from build123d import *

# Parameters (mm, degrees)
SKETCH1_W           = 100
SKETCH1_H           = 200
SKETCH1_W_2         = 67
SKETCH1_H_2         = 110
BOSS_EXTRUDE1_DEPTH = 2
SKETCH2_W           = 100
SKETCH2_H           = 200
SKETCH2_W_2         = 94
SKETCH2_H_2         = 194
BOSS_EXTRUDE2_DEPTH = 16.4
SKETCH3_R           = 1.15
BOSS_EXTRUDE3_DEPTH = 2
BOSS_EXTRUDE4_DEPTH = 25
SKETCH8_W           = 100
SKETCH8_H           = 110
BOSS_EXTRUDE5_DEPTH = 3
SKETCH9_W           = 11
SKETCH9_H           = 13
CUT_EXTRUDE2_DEPTH  = 36
SKETCH13_W          = 141.504865249
SKETCH13_H          = 212.967188503
CUT_EXTRUDE6_DEPTH  = 3.1
SKETCH14_W          = 94
SKETCH14_H          = 194
BOSS_EXTRUDE6_DEPTH = 3
CUT_EXTRUDE7_DEPTH  = 3
SKETCH15_R          = 2
CUT_EXTRUDE8_DEPTH  = 3
SKETCH16_R          = 2
CUT_EXTRUDE9_DEPTH  = 3
SKETCH17_R          = 2
CUT_EXTRUDE10_DEPTH = 3


with BuildPart() as part:
    # Sketch1 → Boss-Extrude1 (new body)
    with BuildSketch(Plane(origin=(0, 0, 0), x_dir=(1, 0, 0), z_dir=(0, 1, 0))):
        Rectangle(SKETCH1_W, SKETCH1_H)
        with Locations((0, 35)):
            Rectangle(SKETCH1_W_2, SKETCH1_H_2, mode=Mode.SUBTRACT)
    extrude(amount=BOSS_EXTRUDE1_DEPTH)

    # Sketch2 → Boss-Extrude2 (add)
    with BuildSketch(Plane.XZ):
        Rectangle(SKETCH2_W, SKETCH2_H)
        Rectangle(SKETCH2_W_2, SKETCH2_H_2, mode=Mode.SUBTRACT)
    extrude(amount=BOSS_EXTRUDE2_DEPTH)

    # Sketch3 → Boss-Extrude3 (add)
    with BuildSketch(Plane.XZ.offset(16.4)):
        Polygon((-50, 100), (50, 100), (50, 10), (50, -11), (30, -11), (30, -1), (35, -1), (35, 10), (35, 80), (-35, 80), (-35, 10), (-35, -1), (-30, -1), (-30, -11), (-50, -11), (-50, 10), align=None)
        with Locations(Location((-35, 85, 0), (0, 0, 270))):
            Circle(SKETCH3_R, mode=Mode.SUBTRACT)
        with Locations(Location((35, 85, 0), (0, 0, 270))):
            Circle(SKETCH3_R, mode=Mode.SUBTRACT)
        with Locations(Location((-35, -6, 0), (0, 0, 270))):
            Circle(SKETCH3_R, mode=Mode.SUBTRACT)
        with Locations(Location((35, -6, 0), (0, 0, 270))):
            Circle(SKETCH3_R, mode=Mode.SUBTRACT)
    extrude(amount=BOSS_EXTRUDE3_DEPTH)

    # Sketch5 → Boss-Extrude4 (add)
    with BuildSketch(Plane.XZ.offset(16.4)):
        Polygon((-50, -100), (50, -100), (50, -97), (50, 10), (47, 10), (47, -97), (-47, -97), (-47, 10), (-50, 10), (-50, -97), align=None)
    extrude(amount=BOSS_EXTRUDE4_DEPTH)

    # Sketch8 → Boss-Extrude5 (add)
    with BuildSketch(Plane.XZ.offset(41.4)):
        with Locations((0, -45)):
            Rectangle(SKETCH8_W, SKETCH8_H)
    extrude(amount=BOSS_EXTRUDE5_DEPTH)

    # Sketch9 → Cut-Extrude2 (cut)
    with BuildSketch(Plane(origin=(0, -16.4, 0), x_dir=(1, 0, 0), z_dir=(0, 1, 0))):
        with Locations((-28.65, -74.5)):
            Rectangle(SKETCH9_W, SKETCH9_H)
        with Locations((-0.71, -74.5)):
            Rectangle(SKETCH9_W, SKETCH9_H)
        with Locations((24.69, -74.5)):
            Rectangle(SKETCH9_W, SKETCH9_H)
        with Locations((-28.65, -49.1)):
            Rectangle(SKETCH9_W, SKETCH9_H)
        with Locations((-0.71, -49.1)):
            Rectangle(SKETCH9_W, SKETCH9_H)
        with Locations((24.69, -49.1)):
            Rectangle(SKETCH9_W, SKETCH9_H)
    extrude(amount=CUT_EXTRUDE2_DEPTH, mode=Mode.SUBTRACT)

    # Sketch13 → Cut-Extrude6 (cut)
    with BuildSketch(Plane(origin=(0, 2, 0), x_dir=(1, 0, 0), z_dir=(0, 1, 0))):
        with Locations((7.572166702, -0.236630209)):
            Rectangle(SKETCH13_W, SKETCH13_H)
    extrude(amount=-CUT_EXTRUDE6_DEPTH, mode=Mode.SUBTRACT)

    # Sketch14 → Boss-Extrude6 (add)
    with BuildSketch(Plane(origin=(0, -1.1, 0), x_dir=(1, 0, 0), z_dir=(0, 1, 0))):
        Rectangle(SKETCH14_W, SKETCH14_H)
    extrude(amount=-BOSS_EXTRUDE6_DEPTH)

    # Sketch14_4 → Cut-Extrude7 (cut)
    with BuildSketch(Plane(origin=(0, -1.1, 0), x_dir=(1, 0, 0), z_dir=(0, 1, 0))):
        Polygon((-32, 92), (32, 92), (32, 82), (42, 82), (42, -25), (32, -25), (32, -40), (42, -40), (42, -82), (32, -82), (32, -92), (-32, -92), (-32, -82), (-42, -82), (-42, -40), (-32, -40), (-32, -25), (-42, -25), (-42, 82), (-32, 82), align=None)
    extrude(amount=-CUT_EXTRUDE7_DEPTH, mode=Mode.SUBTRACT)

    # Sketch15 → Cut-Extrude8 (cut)
    with BuildSketch(Plane.XZ.offset(44.4)):
        with Locations(Location((-40, 0, 0), (0, 0, 270))):
            Circle(SKETCH15_R)
        with Locations(Location((40, 0, 0), (0, 0, 270))):
            Circle(SKETCH15_R)
    extrude(amount=-CUT_EXTRUDE8_DEPTH, mode=Mode.SUBTRACT)

    # Sketch16 → Cut-Extrude9 (cut)
    with BuildSketch(Plane.XZ.offset(18.4)):
        with Locations(Location((-40, 92.5, 0), (0, 0, 270))):
            Circle(SKETCH16_R)
        with Locations(Location((40, 92.5, 0), (0, 0, 270))):
            Circle(SKETCH16_R)
    extrude(amount=-CUT_EXTRUDE9_DEPTH, mode=Mode.SUBTRACT)

    # Sketch17 → Cut-Extrude10 (cut)
    with BuildSketch(Plane(origin=(0, -1.1, 0), x_dir=(1, 0, 0), z_dir=(0, 1, 0))):
        with Locations(Location((-41, 91, 0), (0, 0, 270))):
            Circle(SKETCH17_R)
        with Locations(Location((41, 91, 0), (0, 0, 270))):
            Circle(SKETCH17_R)
        with Locations(Location((-41, -32.5, 0), (0, 0, 270))):
            Circle(SKETCH17_R)
        with Locations(Location((41, -32.5, 0), (0, 0, 270))):
            Circle(SKETCH17_R)
        with Locations(Location((-41, -91, 0), (0, 0, 270))):
            Circle(SKETCH17_R)
        with Locations(Location((41, -91, 0), (0, 0, 270))):
            Circle(SKETCH17_R)
    extrude(amount=-CUT_EXTRUDE10_DEPTH, mode=Mode.SUBTRACT)


solid = part.part
The model under review builds one solid part; all positions refer to its coordinate system, in mm. A direction names the side the tool comes from. Give positions to 0.01 mm unless a question says otherwise; leave off trailing zeros. Write each loop counter-clockwise with the first axis right and the second up, starting at its lowest first coordinate (ties: lowest second). Pieces come first, ordered by that corner, then holes.
1. For P1, Ø5, axis at x = -40, z = 0, coming from the -Y side; P2, Ø3.5, axis at x = -41, z = 32.5, coming from the -Y side; P3, Ø4, axis at y = -22, z = 61.5, coming from the -X side; P4, Ø1.4, axis at x = -35, z = -6, coming from the +Y side, all flat-tipped, find the tip position at first contact; note any pin that passes through.
2. Add section A-A, the plane z = 63. Write out the cut boundary in (x, y).
3. Add section B-B, the plane x = 15.5. Write out the cut boundary in (y, z).
4. Wall thickness on L1, parallel to X at y = -42.9, z = 0; L2, parallel to X at y = -17, z = 85; L3, parallel to Z at x = -12.5, y = -5: over which ranges is each line inside the solid? List them lowest first.
5. Add section C-C, the plane y = -12. Write out the cut boundary in (x, z), plus the area to 3 significant figures.
6. Draft analysis for pull direction Z (two halves, no side actions). For faces 5 (the flat face through (1, -18.4, 82)), 6 (the cylindrical face through (39.234, -17.414, 90.653)), 7 (the flat face through (0, -43, 10)), state which applies: +Z half, -Z half, draft (parallel to the pull), parting line (faces both ways), or undercut.
7. Tool access review of faces 1 (the cylindrical face through (-41.774, -17.414, 91.577)), 2 (the flat face through (1, -22, -97)), 3 (the cylindrical face through (39.226, -2.579, 33.423)), 4 (the flat face through (-1, -41.4, -43)): name each direction out of +Z, -Z, +X, -X, +Y, -Y from which nothing blocks a thin tool from reaching the whole face with its end or side.
8. Add section D-D, the plane z = -26.5. Write out the cut boundary in (x, y).
Worked answers:
1. P1: stops at y = -44.4
1. P2: stops at y = -18.4
1. P3: passes through
1. P4: stops at y = -41.4
2. outline: (-50, -18.4) - (-35, -18.4) - (-35, -16.4) - (-47, -16.4) - (-47, -4.1) - (-42, -4.1) - (-42, -1.1) - (-50, -1.1) - close; (35, -18.4) - (50, -18.4) - (50, -1.1) - (42, -1.1) - (42, -4.1) - (47, -4.1) - (47, -16.4) - (35, -16.4) - close
3. outline: (-44.4, -100) - (-1.1, -100) - (-1.1, -92) - (-4.1, -92) - (-4.1, -97) - (-41.4, -97) - (-41.4, 10) - (-44.4, 10) - close; (-18.4, 80) - (-16.4, 80) - (-16.4, 97) - (-4.1, 97) - (-4.1, 92) - (-1.1, 92) - (-1.1, 100) - (-18.4, 100) - close
4. L1: x = -50 to -42, -38 to 38, 42 to 50
4. L2: x = -50 to -36.15, -33.85 to 33.85, 36.15 to 50
4. L3: z = -100 to -97, 97 to 100
5. outline: (-50, -100) - (50, -100) - (50, 100) - (-50, 100) - close; hole (-47, -97) - (47, -97) - (47, 97) - (-47, 97) - close
5. area: 1,760 mm2
6. face 5: draft
6. face 6: undercut
6. face 7: +Z half
7. face 1: -Y
7. face 2: none
7. face 3: +Y
7. face 4: +Z
8. outline: (-50, -44.4) - (50, -44.4) - (50, -1.1) - (42, -1.1) - (42, -4.1) - (47, -4.1) - (47, -41.4) - (-47, -41.4) - (-47, -4.1) - (-42, -4.1) - (-42, -1.1) - (-50, -1.1) - close
